Verification items for the finished model (mm, model axes). Face numbers are marked on the shaded views. Round coordinates to 2 decimals unless told otherwise and drop trailing zeros. Write each loop counter-clockwise with the first axis right and the second up, starting at its lowest first coordinate (ties: lowest second). Pieces come first, ordered by that corner, then holes. Notation, with made-up numbers: M 50.5,-38 L 84.5,-38 A30 ccw 84.5,0 Z; hole C -38,3 d9. An arc over 180 degrees is marked long. Answer in a Markdown table with one row per item. Add a question column.
1. Sectioned sample at D-D on y = -22.5. Record the cut outline in (x, z), plus the area to 3 significant figures.
2. Material ranges on probe 1 along Z at (x, y) = (9.5, -14); probe 2 along X at (y, z) = (-24, 43); probe 3 along X at (y, z) = (-50, 33), recorded low to high.
3. Sectioned sample at A-A on z = 31. Record the cut outline in (x, y), plus the area to 3 significant figures.
4. Sectioned sample at C-C on x = 9. Record the cut outline in (y, z), plus the area to 3 significant figures.
5. Sectioned sample at B-B on y = -14.5. Record the cut outline in (x, z).
6. Draft check along X on the marked faces 1, 2, 3 and 4. Enter one of: pulls with the +X half, pulls with the -X half, needs draft (parallel to the pull), parting line crosses it, or undercut.
7. Go/stop test with flat-tipped pins: pin 1 Ø12 at (y, z) = (7.5, 45) entering from +X; pin 2 Ø23 at (x, y) = (15.5, -18.5) entering from +Z. Record where each tip stops, or that it passes through.
```python
from build123d import *

# Parameters (mm, degrees)
F0_W     = 101.6
F0_H     = 76.2
F1_DEPTH = 25.4
F5_DEPTH = 25.4
F8_DEPTH = 25.4


# Not quite as in the source:
# - a feature of the source that left no trace in its solid (it failed there, or was rolled back) is left out


with BuildPart() as f1:
    # F0 (on Top) → F1 (new body)
    with BuildSketch(Plane.XY):
        with Locations((-10.3016215888, -18.0514037281)):
            Rectangle(F0_W, F0_H)
    extrude(amount=F1_DEPTH)

    # F4 (on face) → F5 (join)
    with BuildSketch(Plane.XY.offset(25.4)):
        Polygon((15.0983784112, -56.1514037281), (40.4983784112, -56.1514037281), (40.4983784112, -11.0943727195), align=None)
    extrude(amount=F5_DEPTH)

    # F7 (on face) → F8 (join)
    with BuildSketch(Plane.XY.offset(25.4)):
        Polygon((-61.1016215888, -56.1514037281), (-48.4016215888, -56.1514037281), (2.3983784112, 20.0485962719), (-61.1016215888, 20.0485962719), align=None)
    extrude(amount=F8_DEPTH)


solid = f1.part
```
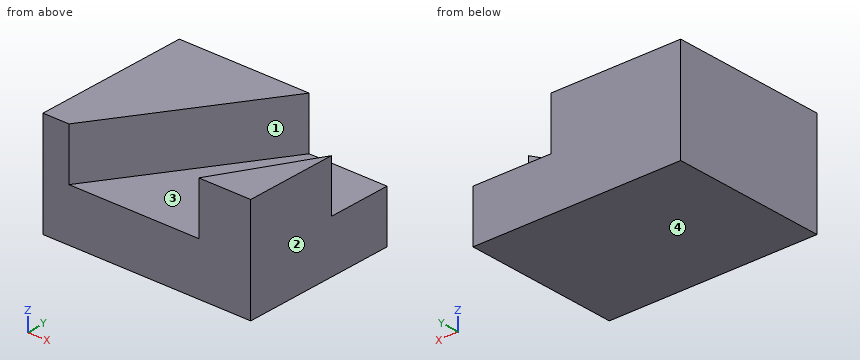
Geometry check:
| question | item | result |
|---|---|---|
| 1 | outline | M -61.1,0 L 40.5,0 L 40.5,50.8 L 34.07,50.8 L 34.07,25.4 L -25.97,25.4 L -25.97,50.8 L -61.1,50.8 Z |
| 1 | area | 3,640 mm2 |
| 2 | probe 1 | z = 0 to 25.4 |
| 2 | probe 2 | x = -61.1 to -26.97, 33.22 to 40.5 |
| 2 | probe 3 | x = -61.1 to -44.3, 18.57 to 40.5 |
| 3 | outline | M -61.1,-56.15 L -48.4,-56.15 L 2.4,20.05 L -61.1,20.05 Z; M 15.1,-56.15 L 40.5,-56.15 L 40.5,-11.09 Z |
| 3 | area | 3,480 mm2 |
| 4 | outline | M -56.15,0 L 20.05,0 L 20.05,25.4 L -56.15,25.4 Z |
| 4 | area | 1,940 mm2 |
| 5 | outline | M -61.1,0 L 40.5,0 L 40.5,50.8 L 38.58,50.8 L 38.58,25.4 L -20.63,25.4 L -20.63,50.8 L -61.1,50.8 Z |
| 6 | face 1 | undercut |
| 6 | face 2 | pulls with the +X half |
| 6 | face 3 | undercut |
| 6 | face 4 | needs draft |
| 7 | pin 1 | stops at x = -1.97 |
| 7 | pin 2 | stops at z = 25.4 |
